Read the model definition and answer for the solid it produces. Units are mm, in the model's axes. Round coordinates to 2 decimals unless told otherwise and drop trailing zeros. Write each loop counter-clockwise with the first axis right and the second up, starting at its lowest first coordinate (ties: lowest second). Pieces come first, ordered by that corner, then holes.
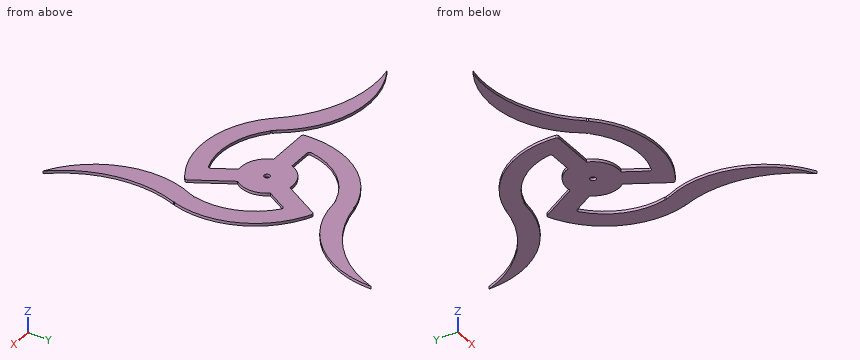
from build123d import *

# Parameters (mm, degrees)
F2_DEPTH        = 1.524
F0_R            = 14.2875
F0_R_2          = 1.5875
F3_COUNT        = 3
F3_ANGLE        = 240
F6_DEPTH        = 240
F6_COPIES_COUNT = 3


# Not quite as in the source:
# - an extrude ends at something that could not be found from the text; its depth is read off the source's solid
# - a pattern or mirror of a feature is missing from the dataset's text; its kind, count and spacing are read off the source's solid
# - a feature names something its author has since deleted; it is built from what else it names


with BuildPart() as f2:
    # F0 (on Top) → F2 (new body)
    with BuildSketch(Plane.XY):
        with BuildLine():
            ThreePointArc((50.8, 90.4875), (31.2220900836, 62.3697318544), (0, 48.26))
            ThreePointArc((0, 48.26), (-27.5567729007, 30.8458733427), (-38.1, 0))
            Line((-38.1, 0), (-27.9404663148, 0.0973411457))
            ThreePointArc((-27.9404663148, 0.0973411457), (-19.5823640029, 24.5502873707), (2.2631606282, 38.3552686068))
            ThreePointArc((2.2631606282, 38.3552686068), (36.7873562722, 54.8729161676), (50.8, 90.4875))
        make_face()
    extrude(amount=F2_DEPTH)


with BuildPart() as f2b:
    # F0 (on Top) → F2, piece 2 (new body)
    with BuildSketch(Plane.XY):
        Circle(F0_R)
        Circle(F0_R_2, mode=Mode.SUBTRACT)
    extrude(amount=F2_DEPTH)


with BuildPart() as f2c:
    # F1 (on face) → F2, piece 3 (new body)
    with BuildSketch(Plane.XY):
        with BuildLine():
            ThreePointArc((-13.3538854365, -5.08), (-14.2875, 0), (-13.3538854365, 5.08))
            Line((-13.3538854365, 5.08), (-26.2094863625, 5.08))
            ThreePointArc((-26.2094863625, 5.08), (-27.1751979909, 5.5251963562), (-27.4638524569, 6.5486597626))
            ThreePointArc((-27.4638524569, 6.5486597626), (-27.8366270568, 3.3329347264), (-27.9404663148, 0.0973411457))
            Line((-27.9404663148, 0.0973411457), (-38.1, 0))
            ThreePointArc((-38.1, 0), (-38.0418102628, -1.963864994), (-37.9049743558, -3.923821038))
            ThreePointArc((-37.9049743558, -3.923821038), (-37.4969244549, -4.7474040533), (-36.6400851229, -5.08))
            Line((-36.6400851229, -5.08), (-13.3538854365, -5.08))
        make_face()
    extrude(amount=F2_DEPTH)


with BuildPart() as f3_1:
    # F3: instance of F2
    add(f2.part.rotate(Axis((0, 0, 0), (0, 0, 1)), 1 * F3_ANGLE / (F3_COUNT - 1)))


with BuildPart() as f3_2:
    # F3: instance of F2
    add(f2.part.rotate(Axis((0, 0, 0), (0, 0, 1)), 2 * F3_ANGLE / (F3_COUNT - 1)))


with BuildPart() as f3_3:
    # F3: instance of F2c
    add(f2c.part.rotate(Axis((0, 0, 0), (0, 0, 1)), 1 * F3_ANGLE / (F3_COUNT - 1)))


with BuildPart() as f3_4:
    # F3: instance of F2c
    add(f2c.part.rotate(Axis((0, 0, 0), (0, 0, 1)), 2 * F3_ANGLE / (F3_COUNT - 1)))


with BuildPart() as f2_1:
    add(f2.part)

    # F4: union F2c, F2b, F3_4, F3_2, F3_3, F3_1
    add(f2c.part)
    add(f2b.part)
    add(f3_4.part)
    add(f3_2.part)
    add(f3_3.part)
    add(f3_1.part)

    # F5 (on face) → F6 (cut, through all)
    with BuildSketch(Plane.XY.offset(1.524)):
        with BuildLine():
            ThreePointArc((0, 48.26), (0.1881613405, 48.2897596913), (0.3762338884, 48.3200754628))
            ThreePointArc((0.3762338884, 48.3200754628), (-0.0732384475, 48.6338945437), (-0.3710948228, 48.1736887464))
            ThreePointArc((-0.3710948228, 48.1736887464), (-0.1856312633, 48.2172048941), (0, 48.26))
        make_face()
        with BuildLine():
            ThreePointArc((-0.3710948228, 48.1736887464), (0.0434388796, 47.8814843943), (0.381, 48.26))
            ThreePointArc((0.381, 48.26), (0.3798066031, 48.2901321135), (0.3762338884, 48.3200754628))
            ThreePointArc((0.3762338884, 48.3200754628), (0.1881613405, 48.2897596913), (0, 48.26))
            ThreePointArc((0, 48.26), (-0.1856312633, 48.2172048941), (-0.3710948228, 48.1736887464))
        make_face()
        with BuildLine():
            ThreePointArc((-0.3651208351, 37.6571250082), (0, 37.7659724968), (0.3661704074, 37.8712351814))
            ThreePointArc((0.3661704074, 37.8712351814), (-0.1070563729, 38.1316225112), (-0.3651208351, 37.6571250082))
        make_face()
    f6 = extrude(amount=-F6_DEPTH, mode=Mode.SUBTRACT)

    # F6_copies: F6 ×3 about axis
    f6_copies_axis = Axis((0, 0, 0), (0, 0, 1))
    for i in range(1, F6_COPIES_COUNT):
        add(f6.rotate(f6_copies_axis, i * 360 / F6_COPIES_COUNT), mode=Mode.SUBTRACT)


solid = f2_1.part
Q1. Section A-A (x = -50) is taken. Determine the outline of the cut face in (y, z).
Verdict:
outline: (-15.68, 0) - (-2.15, 0) - (-2.15, 1.52) - (-15.68, 1.52) - close
Q2. Straight lines are drawn through the part: probe 1 along Y at (x, z) = (0, 1); probe 2 along Y at (x, z) = (-17, 1); probe 3 along Y at (x, z) = (-18.5, 1.3). For each, find the intervals that lie inside material, in ascending order.
Verdict:
probe 1: y = -39.45 to -29.19, -14.29 to -1.59, 1.59 to 14.29, 38.15 to 47.88
probe 2: y = -38.52 to -28.01, -5.08 to 5.08, 27.5 to 40.76
probe 3: y = -38.14 to -27.53, -5.08 to 5.08, 25.86 to 39.68
Q3. A flat-ended cylindrical pin translates along its axis: pin 1 Ø3 at (x, y) = (0, 0) entering from +Z. Find the tip coordinate at first contact, or state that the pin passes through.
Verdict:
pin 1: passes through
Q4. Section B-B (y = 59.5) is taken. Determine the outline of the cut face in (x, z), then the cut area to 3 significant figures.
Verdict:
outline: (27.5, 0) - (40.62, 0) - (40.62, 1.52) - (27.5, 1.52) - close
area: 20.0 mm2
